Part print with two shaded views. Sizes in mm from the minimum x, y, z corner. A direction names the side the tool comes from. Coordinates: 2 decimals unless noted, no trailing zeros. Loops run counter-clockwise (first coordinate to the right, second up) from the corner with the lowest first, then second, coordinate; pieces in that order, holes last. Notation, with made-up numbers: (48.5, 27) -> (61.5, 27) arc R33 cw to (61.5, 61) -> close; hole circle Ø4 at (21.25, -18.5). An arc over 180 degrees is marked (long way). Return JSON: item names as keys, results as strings. Group by question number.
(1) Probe L1, parallel to Y at x = 25, z = 6.25; L2, parallel to Y at x = 25, z = 15.25; L3, parallel to Z at x = 43, y = 6.5. List the from-to ranges inside material, lowest first.
(2) Tool access for the marked faces 5 and 6: list every direction of +Z, -Z, +X, -X, +Y, -Y with a clear straight run to the whole face (end or side of a thin tool).
(3) Mould opens along Y. For the marked faces 1, 2, 3 and 4 say: pulls with the +Y half, pulls with the -Y half, needs draft (parallel to the pull), parting line crosses it, or undercut.
(4) Flat gauge pins, fed straight in: pin 1 Ø7.5 at (x, z) = (24, 11.5) entering from +Y; pin 2 Ø2.5 at (x, z) = (31.5, 18) entering from -Y; pin 3 Ø5.5 at (x, y) = (21, 2.5) entering from +Z. Where does each tip first touch, or does it go through?
(5) Saw through at B-B on y = 25. Write the cut outline in (x, z), then the cut area to 3 significant figures.
(6) Saw through at D-D on x = 38. Write the cut outline in (y, z), then the cut area to 3 significant figures.
(7) Saw through at A-A on x = 25. Write the cut outline in (y, z), then the cut area to 3 significant figures.
(8) Saw through at C-C on z = 11.5. Write the cut outline in (x, y).
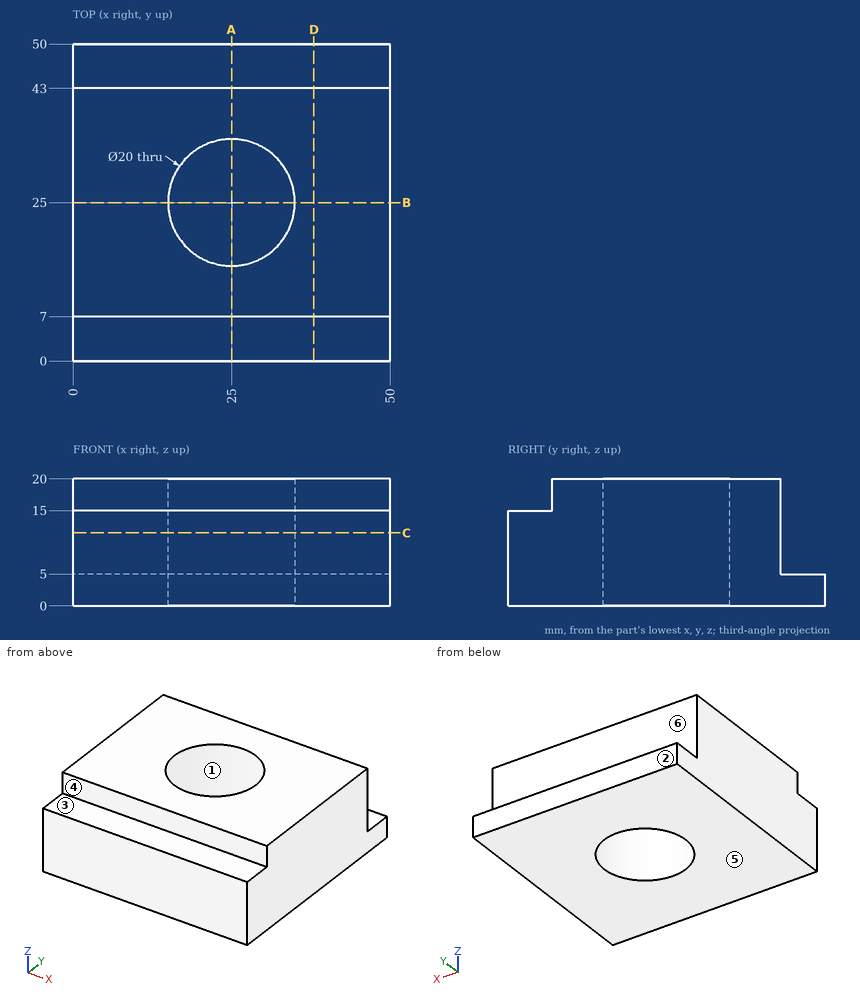
Geometry results:
{
 "1": {"L1": "0 to 15, 35 to 43", "L2": "7 to 15, 35 to 43", "L3": "0 to 15"},
 "2": {"face 5": "-Z, +X, -X, +Y, -Y", "face 6": "+Z, +X, -X, +Y"},
 "3": {"face 1": "undercut", "face 2": "pulls with the +Y half", "face 3": "needs draft", "face 4": "pulls with the -Y half"},
 "4": {"pin 1": "y = 43", "pin 2": "y = 7", "pin 3": "z = 15"},
 "5": {"outline": "(0, 0) -> (15, 0) -> (15, 20) -> (0, 20) -> close; (35, 0) -> (50, 0) -> (50, 20) -> (35, 20) -> close", "area": "600 mm²"},
 "6": {"outline": "(0, 0) -> (50, 0) -> (50, 5) -> (43, 5) -> (43, 20) -> (7, 20) -> (7, 15) -> (0, 15) -> close", "area": "860 mm²"},
 "7": {"outline": "(0, 0) -> (15, 0) -> (15, 20) -> (7, 20) -> (7, 15) -> (0, 15) -> close; (35, 0) -> (50, 0) -> (50, 5) -> (43, 5) -> (43, 20) -> (35, 20) -> close", "area": "460 mm²"},
 "8": {"outline": "(0, 0) -> (50, 0) -> (50, 43) -> (0, 43) -> close; hole circle Ø20 at (25, 25)"}
}
